Source: CAD feature listing. Evaluate the final solid. Frame: model axes, mm. A direction names the side the tool comes from. Give positions to 0.01 mm unless a question says otherwise; leave off trailing zeros. Order: outer loops, then holes, each group sorted by start corner. A loop starts at its lowest first (then second) coordinate and runs counter-clockwise, first axis right, second up. Notation, with made-up numbers: (-27.5, -10) -> (-15.5, -10) arc R24 ccw to (-15.5, 10) -> close; hole circle Ø10 at (-14.5, 17). An arc over 180 degrees is marked (long way). Use one line per item in the form item = value. Start each with the question number.
from build123d import *

# Parameters (mm, degrees)
SKETCH1_R           = 1.25
BOSS_EXTRUDE1_DEPTH = 3.175
BOSS_EXTRUDE2_DEPTH = 3.175
BOSS_EXTRUDE3_DEPTH = 42.2
BOSS_EXTRUDE4_DEPTH = 3.175


with BuildPart() as part:
    # Sketch1 → Boss-Extrude1 (new body)
    with BuildSketch(Plane(origin=(0, 90.055223859, 0), x_dir=(1, 0, 0), z_dir=(0, 1, 0))):
        Polygon((-138.728927309, 21.91435009), (-167.073938775, 38.27935009), (-179.573938775, 16.628714996), (-151.228927309, 0.263714996), align=None)
        with Locations((-169.089659252, 19.059098981)):
            Circle(SKETCH1_R, mode=Mode.SUBTRACT)
        with Locations((-162.879788078, 29.814911363)):
            Circle(SKETCH1_R, mode=Mode.SUBTRACT)
        with Locations((-153.337652818, 21.865216105)):
            Circle(SKETCH1_R, mode=Mode.SUBTRACT)
        with Locations((-159.547523992, 11.109403723)):
            Circle(SKETCH1_R, mode=Mode.SUBTRACT)
    extrude(amount=BOSS_EXTRUDE1_DEPTH)

    # Sketch2 → Boss-Extrude2 (add)
    with BuildSketch(Plane(origin=(0, 93.230223859, 0), x_dir=(1, 0, 0), z_dir=(0, 1, 0))):
        with BuildLine():
            Line((-161.213656035, 20.462157543), (-237.413656035, 152.44442908))
            ThreePointArc((-237.413656035, 152.44442908), (-293.195927572, 96.662157543), (-313.613656035, 20.462157543))
            Line((-313.613656035, 20.462157543), (-161.213656035, 20.462157543))
        make_face()
        with BuildLine():
            Line((-166.712917349, 23.637157543), (-238.558896482, 148.078043722))
            ThreePointArc((-238.558896482, 148.078043722), (-290.446296915, 95.074657543), (-310.404875616, 23.637157543))
            Line((-310.404875616, 23.637157543), (-166.712917349, 23.637157543))
        make_face(mode=Mode.SUBTRACT)
    extrude(amount=-BOSS_EXTRUDE2_DEPTH)

    # Sketch3 → Boss-Extrude3 (add)
    with BuildSketch(Plane(origin=(0, 93.230223859, 0), x_dir=(1, 0, 0), z_dir=(0, 1, 0))):
        with BuildLine():
            Line((-238.558896482, 148.078043722), (-240.204539896, 150.793275343))
            ThreePointArc((-240.204539896, 150.793275343), (-238.813489705, 151.626275405), (-237.413656035, 152.44442908))
            Line((-237.413656035, 152.44442908), (-235.809265825, 149.665543722))
            Line((-235.809265825, 149.665543722), (-238.558896482, 148.078043722))
        make_face()
        with BuildLine():
            Line((-310.404875616, 20.462157543), (-313.613656035, 20.462157543))
            ThreePointArc((-313.613656035, 20.462157543), (-313.605031003, 22.0835259), (-313.579156883, 23.704710735))
            Line((-313.579156883, 23.704710735), (-310.404875616, 23.637157543))
            Line((-310.404875616, 23.637157543), (-310.404875616, 20.462157543))
        make_face()
        with BuildLine():
            Line((-277.541611418, 113.928233857), (-280.016674298, 115.916873778))
            ThreePointArc((-280.016674298, 115.916873778), (-278.994417499, 117.175404976), (-277.958829166, 118.422989259))
            Line((-277.958829166, 118.422989259), (-275.500760757, 116.360424964))
            Line((-275.500760757, 116.360424964), (-277.541611418, 113.928233857))
        make_face()
        with BuildLine():
            Line((-302.493458116, 68.505035776), (-305.499411352, 69.527224675))
            ThreePointArc((-305.499411352, 69.527224675), (-304.969247202, 71.059489571), (-304.422811443, 72.586027386))
            Line((-304.422811443, 72.586027386), (-301.407544161, 71.488559847))
            Line((-301.407544161, 71.488559847), (-302.493458116, 68.505035776))
        make_face()
    extrude(amount=BOSS_EXTRUDE3_DEPTH)

    # Sketch4 → Boss-Extrude4 (add)
    with BuildSketch(Plane(origin=(0, 135.430223859, 0), x_dir=(1, 0, 0), z_dir=(0, 1, 0))):
        with BuildLine():
            Line((-237.413656035, 152.44442908), (-235.809265825, 149.665543722))
            ThreePointArc((-235.809265825, 149.665543722), (-290.417042213, 95.057767334), (-310.404875616, 20.462157543))
            Line((-310.404875616, 20.462157543), (-313.613656035, 20.462157543))
            ThreePointArc((-313.613656035, 20.462157543), (-293.195927572, 96.662157543), (-237.413656035, 152.44442908))
        make_face()
    extrude(amount=BOSS_EXTRUDE4_DEPTH)


solid = part.part
1) Draft query along Y for faces 1 (the face through (-258, 135.43, -135)), 2 (the face through (-152.7, 91.62, -29.98)), 3 (the face through (-292, 138.605, -97)). Return one class per face: +Y half, -Y half, draft (parallel to the pull), parting line (faces both ways), or undercut.
2) Cut plane C-C, the plane y = 96. Return the cut outline in (x, z).
3) Cut plane A-A, the plane x = -285.5. Return the cut outline in (y, z), plus the area to 3 significant figures.
4) Pin query (flat end, axial travel): pin 1 (10 mm diameter, centred on y = 127, z = -18, fed in from +X); pin 2 (3 mm diameter, centred on x = -169.09, z = -19.06, fed in from +Y); pin 3 (12 mm diameter, centred on x = -270.5, y = 127, fed in from -Z). Return the tip coordinate at first contact, or that it passes through.
5) Cut plane D-D, the plane x = -210. Return the cut outline in (y, z), plus the area to 3 significant figures.
6) Reachability of faces 4 (the face through (-194.2, 90.055, -76.7)), 5 (the face through (-173.29, 91.62, -27.51)) from +Z, -Z, +X, -X, +Y, -Y: full face, straight path, thin tool, end or side. Return the list, or none.
7) Material intervals for probe 1 along X at (y, z) = (108, -22); probe 2 along X at (y, z) = (92.5, -10.5); probe 3 along Y at (x, z) = (-156.5, -25), sorted ascending.
8) Cut plane B-B, the plane z = -48. Return the cut outline in (x, y).
Output values:
q1.face_1 = undercut
q1.face_2 = draft
q1.face_3 = +Y half
q2.outline = (-313.61, -20.46) arc R152.4 ccw to (-313.58, -23.7) -> (-310.4, -23.64) -> (-310.4, -20.46) -> close; (-305.5, -69.53) arc R152.4 ccw to (-304.42, -72.59) -> (-301.41, -71.49) -> (-302.49, -68.51) -> close; (-280.02, -115.92) arc R152.4 ccw to (-277.96, -118.42) -> (-275.5, -116.36) -> (-277.54, -113.93) -> close; (-240.2, -150.79) arc R152.4 ccw to (-237.41, -152.44) -> (-235.81, -149.67) -> (-238.56, -148.08) -> close
q3.outline = (90.06, -108.66) -> (93.23, -108.66) -> (93.23, -103.05) -> (90.06, -103.05) -> close; (90.06, -23.64) -> (93.23, -23.64) -> (93.23, -20.46) -> (90.06, -20.46) -> close; (135.43, -108.66) -> (138.61, -108.66) -> (138.61, -102.99) -> (135.43, -102.99) -> close
q3.area = 45.9 mm^2
q4.pin_1 = -310.4
q4.pin_2 = 93.23
q4.pin_3 = -117.2
q5.outline = (90.06, -104.96) -> (93.23, -104.96) -> (93.23, -98.61) -> (90.06, -98.61) -> close; (90.06, -23.64) -> (93.23, -23.64) -> (93.23, -20.46) -> (90.06, -20.46) -> close
q5.area = 30.2 mm^2
q6.face_4 = +Z, -Z, +X, -X, -Y
q6.face_5 = +Y, -Y
q7.probe_1 = -313.61 to -310.4
q7.probe_2 = -168.96 to -160.64, -158.46 to -145.32
q7.probe_3 = 90.06 to 93.23
q8.outline = (-311.11, 90.06) -> (-307.88, 90.06) -> (-307.88, 93.23) -> (-311.11, 93.23) -> close; (-311.11, 135.43) -> (-307.84, 135.43) -> (-307.84, 138.61) -> (-311.11, 138.61) -> close; (-180.78, 90.06) -> (-177.11, 90.06) -> (-177.11, 93.23) -> (-180.78, 93.23) -> close
